The drawing under review shows one solid part. Ordinate dimensions are in mm from its lowest x, y, z. A direction names the side the tool comes from. Round coordinates to 2 decimals unless told otherwise and drop trailing zeros. Order: outer loops, then holes, each group sorted by start corner. A loop starts at its lowest first (then second) coordinate and runs counter-clockwise, first axis right, second up. Notation, with made-up numbers: (57.5, -30.5) -> (115.5, -30.5) arc R19 cw to (115.5, -6.5) -> close; hole circle Ø1 at (51, 63.5). An arc over 180 degrees is marked (long way). Put each result on its own line as item: value. Start each with the question number.
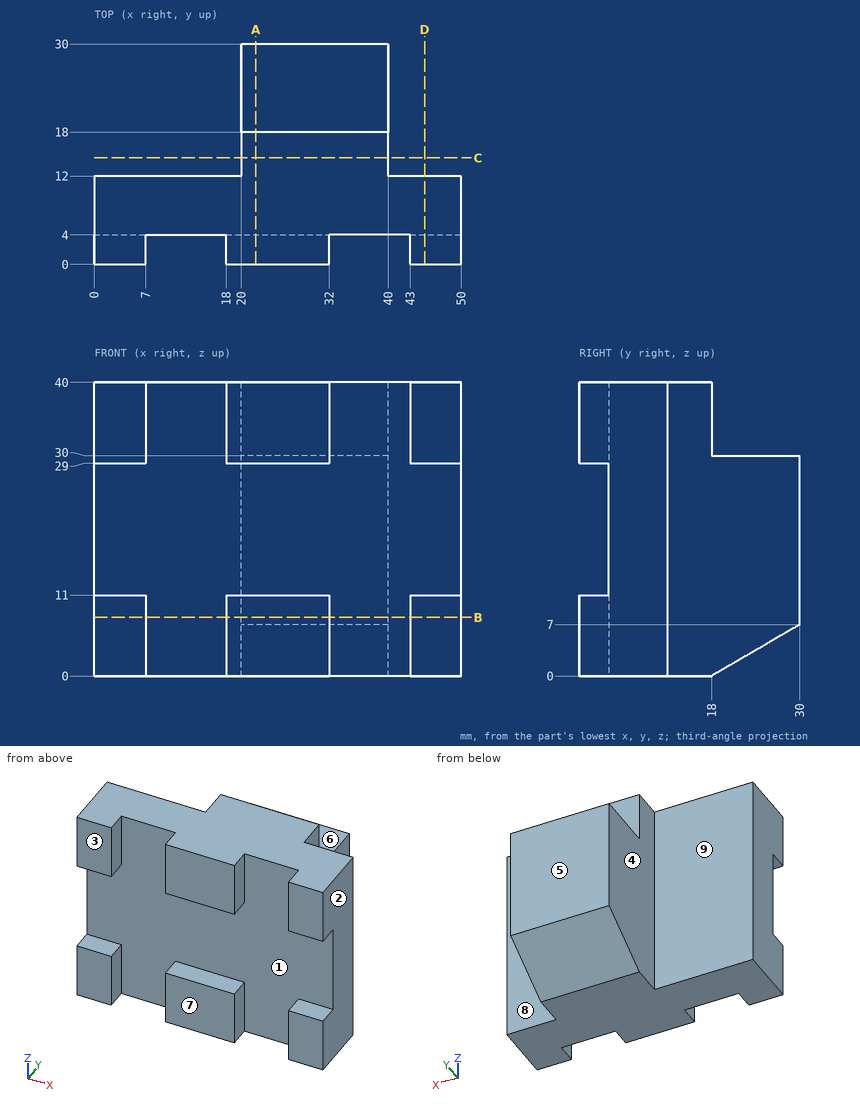
Item 1: Consider section C-C, the plane y = 14.5. Write out the cut boundary in (x, z).
Item 2: Insertion check: pin 1 Ø3.5 at (x, y) = (32.5, 25.5) entering from +Z; pin 2 Ø3 at (y, z) = (17, 4) entering from -X; pin 3 Ø2 at (x, z) = (44, 22) entering from +Y. Each pin has a flat end and moves straight along its axis. Give the tip position at first contact, or say it passes through.
Item 3: Consider section B-B, the plane z = 8. Write out the cut boundary in (x, y).
Item 4: Tool access review of the marked faces 5, 6, 7, 8 and 9: name each direction out of +Z, -Z, +X, -X, +Y, -Y from which nothing blocks a thin tool from reaching the whole face with its end or side.
Item 5: Consider section A-A, the plane x = 22. Write out the cut boundary in (y, z), plus the area to 3 significant figures.
Item 6: For L1, parallel to Y at x = 12, z = 13; L2, parallel to Y at x = 5, z = 9; L3, parallel to X at y = 26.75, z = 28, list the stretches that pass through material, from the lowest coordinate up.
Item 7: Mouldability with a two-part tool opening along X and no side actions: class the marked faces 1, 2, 3 and 4 as +X half, -X half, draft (parallel to the pull), parting line (faces both ways), or undercut.
Item 8: Consider section D-D, the plane x = 45. Write out the cut boundary in (y, z).
Evaluation:
1. outline: (20, 0) -> (40, 0) -> (40, 40) -> (20, 40) -> close
2. pin 1: stops at z = 30
2. pin 2: stops at x = 20
2. pin 3: stops at y = 12
3. outline: (0, 0) -> (7, 0) -> (7, 4) -> (18, 4) -> (18, 0) -> (32, 0) -> (32, 4) -> (43, 4) -> (43, 0) -> (50, 0) -> (50, 12) -> (40, 12) -> (40, 30) -> (20, 30) -> (20, 12) -> (0, 12) -> close
4. face 5: +Z, -Z, +X, -X, +Y
4. face 6: +Z, +X, -X, +Y
4. face 7: +Z, -Z, +X, -X, -Y
4. face 8: +Z, -Z, +X, +Y
4. face 9: +Z, -Z, -X, +Y
5. outline: (0, 0) -> (18, 0) -> (30, 7) -> (30, 30) -> (18, 30) -> (18, 40) -> (0, 40) -> (0, 29) -> (4, 29) -> (4, 11) -> (0, 11) -> close
5. area: 966 mm^2
6. L1: y = 4 to 12
6. L2: y = 0 to 12
6. L3: x = 20 to 40
7. face 1: undercut
7. face 2: +X half
7. face 3: draft
7. face 4: -X half
8. outline: (0, 0) -> (12, 0) -> (12, 40) -> (0, 40) -> (0, 29) -> (4, 29) -> (4, 11) -> (0, 11) -> close
